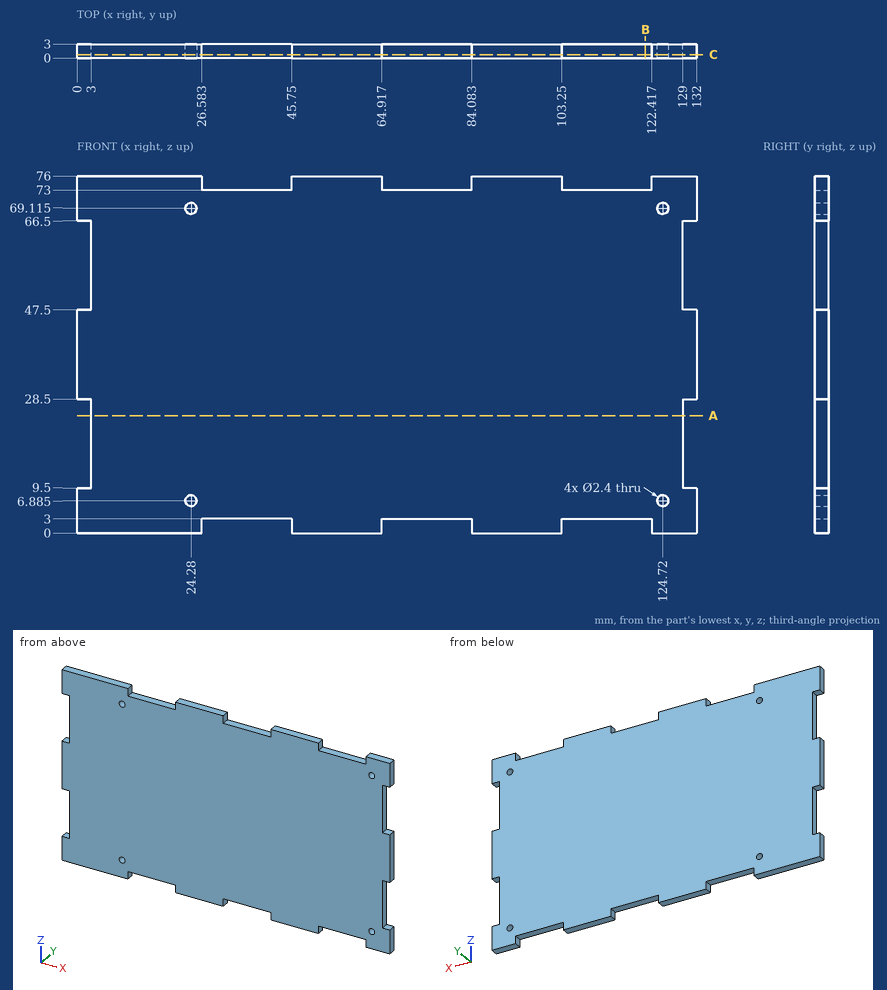
Job drawing, mm, ordinate dimensions from the low corner. One solid piece. Give positions to 0.01 mm unless a question says otherwise; leave off trailing zeros. Write each loop counter-clockwise with the first axis right and the second up, starting at its lowest first coordinate (ties: lowest second). Pieces come first, ordered by that corner, then holes. Notation, with made-up numbers: M 40,-5.75 L 66,-5.75 A28 cw 66,14.25 Z; hole C 77.5,-0.75 d7. An arc over 180 degrees is marked long. One line per item, written item: value. Start each with the question number.
Q1. Saw through at A-A, the plane z = 25. Write the cut outline in (x, y), plus the area to 3 significant figures.
Q2. Saw through at B-B, the plane x = 121. Write the cut outline in (y, z).
Q3. Saw through at C-C, the plane y = 0.75. State how many separate pieces and enclosed holes the cut face has, plus the area to 3 significant figures.
Q4. Drop flat-ended pins along their axis: pin 1 Ø2 at (x, z) = (24.28, 69.115) entering from -Y; pin 2 Ø0.9 at (y, z) = (2, 54.5) entering from -X; pin 3 Ø0.9 at (x, y) = (40.5, 1.5) entering from -Z; pin 4 Ø1.5 at (y, z) = (1.5, 54) entering from +X. Give the stop position or say it passes through.
Q5. Probe probe 1 along Z at (x, y) = (24.28, 1.6) (1 decimal); probe 2 along X at (y, z) = (2.4, 13); probe 3 along Z at (x, y) = (77.5, 1). List the from-to ranges inside material, lowest first. Write a range as [from, to].
Output values:
1. outline: M 3,0 L 129,0 L 129,3 L 3,3 Z
1. area: 378 mm²
2. outline: M 0,3 L 3,3 L 3,73 L 0,73 Z
3. separate pieces: 1
3. enclosed holes: 4
3. area: 9,440 mm²
4. pin 1: passes through
4. pin 2: stops at x = 3
4. pin 3: stops at z = 3
4. pin 4: stops at x = 129
5. probe 1: z = [0, 5.7], [8.1, 67.9], [70.3, 76]
5. probe 2: x = [3, 129]
5. probe 3: z = [3, 73]
